CAD build for the part. Positions are in the model's coordinates, mm. A direction names the side the tool comes from. Round coordinates to 2 decimals unless told otherwise and drop trailing zeros. Loops run counter-clockwise (first coordinate to the right, second up) from the corner with the lowest first, then second, coordinate; pieces in that order, holes last. Notation, with made-up numbers: (46, -17.75) - (104, -17.75) arc R23 ccw to (104, 17.25) - close; hole circle Ø5 at (79.5, 59). An arc over 180 degrees is marked (long way). One line per question, with ' | ' between items.
```python
from build123d import *

# Parameters (mm, degrees)
F1_DEPTH        = 20
F2_DEPTH        = 8
F3_DEPTH        = 20
F4_R            = 5
F6_D            = 5.5
F7_R            = 5
F8_W            = 24.5
F8_H            = 5
F9_DEPTH        = 25
F11_D           = 5.5
F11_DEPTH       = 12
F11_CBORE_D     = 9.75
F11_CBORE_DEPTH = 2
F11_TIP         = 1.6523667023


with BuildPart() as f1:
    # F0 (on Top) → F1 (new body)
    with BuildSketch(Plane.XY):
        with BuildLine():
            Line((-7.3353787871, 29.9999998754), (-7.3353787871, 29.0893831246))
            ThreePointArc((-7.3353787871, 29.0893831246), (-23.6649673064, 18.4382568295), (-29.9999998754, 0))
            ThreePointArc((-29.9999998754, 0), (-21.2132033475, -21.2132033475), (0, -29.9999998754))
            ThreePointArc((0, -29.9999998754), (29.7714752963, -3.6958424215), (7.3353787871, 29.0893831246))
            Line((7.3353787871, 29.0893831246), (7.3353787871, 44.0893831246))
            Line((7.3353787871, 44.0893831246), (3.6676893936, 44.0893831246))
            Line((3.6676893936, 44.0893831246), (3.6676893936, 24.7294976599))
            ThreePointArc((3.6676893936, 24.7294976599), (0, -25), (-3.6676893936, 24.7294976599))
            Line((-3.6676893936, 24.7294976599), (-3.6676893936, 44.0893831246))
            Line((-3.6676893936, 44.0893831246), (-7.3353787871, 44.0893831246))
            Line((-7.3353787871, 44.0893831246), (-7.3353787871, 29.9999998754))
        make_face()
    extrude(amount=F1_DEPTH)

    # F0 (on Top) → F2 (join)
    with BuildSketch(Plane.XY):
        with BuildLine():
            Line((-7.3353787871, 29.9999998754), (-7.3353787871, 29.0893831246))
            ThreePointArc((-7.3353787871, 29.0893831246), (-23.6649673064, 18.4382568295), (-29.9999998754, 0))
            ThreePointArc((-29.9999998754, 0), (-21.2132033475, -21.2132033475), (0, -29.9999998754))
            ThreePointArc((0, -29.9999998754), (29.7714752963, -3.6958424215), (7.3353787871, 29.0893831246))
            Line((7.3353787871, 29.0893831246), (7.3353787871, 44.0893831246))
            Line((7.3353787871, 44.0893831246), (3.6676893936, 44.0893831246))
            Line((3.6676893936, 44.0893831246), (3.6676893936, 24.7294976599))
            ThreePointArc((3.6676893936, 24.7294976599), (0, -25), (-3.6676893936, 24.7294976599))
            Line((-3.6676893936, 24.7294976599), (-3.6676893936, 44.0893831246))
            Line((-3.6676893936, 44.0893831246), (-7.3353787871, 44.0893831246))
            Line((-7.3353787871, 44.0893831246), (-7.3353787871, 29.9999998754))
        make_face()
        with BuildLine():
            ThreePointArc((-29.9999998754, 0), (-23.6649673064, 18.4382568295), (-7.3353787871, 29.0893831246))
            Line((-7.3353787871, 29.0893831246), (-7.3353787871, 29.9999998754))
            Line((-7.3353787871, 29.9999998754), (-94.3353787871, 29.9999998754))
            ThreePointArc((-94.3353787871, 29.9999998754), (-96.4566991307, 29.1213202189), (-97.3353787871, 26.9999998754))
            Line((-97.3353787871, 26.9999998754), (-97.3353787871, -26.9999998754))
            ThreePointArc((-97.3353787871, -26.9999998754), (-96.4566991307, -29.1213202189), (-94.3353787871, -29.9999998754))
            Line((-94.3353787871, -29.9999998754), (-42.1122722328, -29.9999998754))
            Line((-42.1122722328, -29.9999998754), (-42.1122722328, 0))
            Line((-42.1122722328, 0), (-29.9999998754, 0))
        make_face()
        with BuildLine():
            ThreePointArc((0, -29.9999998754), (-21.2132033475, -21.2132033475), (-29.9999998754, 0))
            Line((-29.9999998754, 0), (-42.1122722328, 0))
            Line((-42.1122722328, 0), (-42.1122722328, -29.9999998754))
            Line((-42.1122722328, -29.9999998754), (0, -29.9999998754))
        make_face()
    extrude(amount=F2_DEPTH)

    # F0 (on Top) → F3 (join)
    with BuildSketch(Plane.XY):
        with BuildLine():
            ThreePointArc((0, -29.9999998754), (-21.2132033475, -21.2132033475), (-29.9999998754, 0))
            Line((-29.9999998754, 0), (-42.1122722328, 0))
            Line((-42.1122722328, 0), (-42.1122722328, -29.9999998754))
            Line((-42.1122722328, -29.9999998754), (0, -29.9999998754))
        make_face()
    extrude(amount=F3_DEPTH)

    # F4
    f4_edges = [f1.edges().sort_by_distance(p)[0] for p in [
        (5.501534, 44.089383, 0),
        (-5.501534, 44.089383, 0),
        (-5.501534, 44.089383, 20),
        (5.501534, 44.089383, 20),
    ]]
    fillet(f4_edges, radius=F4_R)

    # F6 (through all)
    with Locations(Plane.YZ.offset(7.3353787871)):
        with Locations((35.7856750488, 10)):
            Hole(F6_D / 2)

    # F7
    f7_edges = [f1.edges().sort_by_distance(p)[0] for p in [
        (-42.112272, 0, 14),
        (-30, 0, 14),
    ]]
    fillet(f7_edges, radius=F7_R)

    # F8 (on face) → F9 (cut)
    with BuildSketch(Plane(origin=(0, 0, 0), x_dir=(1, 0, 0), z_dir=(0, 0, -1))):
        with Locations((-28, 23.4999998754)):
            Rectangle(F8_W, F8_H)
    extrude(amount=-F9_DEPTH, mode=Mode.SUBTRACT)

    # F11
    with Locations(Plane.XZ.offset(29.9999998754)):
        with Locations((-35.5, 15), (-20.5, 15)):
            CounterBoreHole(F11_D / 2, F11_CBORE_D / 2, F11_CBORE_DEPTH, depth=F11_DEPTH)
            with Locations((0, 0, -(F11_DEPTH + F11_TIP / 2))):  # 118° drill point
                Cone(0, F11_D / 2, F11_TIP, mode=Mode.SUBTRACT)


solid = f1.part
```
(1) Cut at B-B, the plane x = 15. Write the cut outline in (y, z), then the cut area to 3 significant figures.
Results found:
outline: (-25.98, 0) - (-20, 0) - (-20, 20) - (-25.98, 20) - close; (20, 0) - (25.98, 0) - (25.98, 20) - (20, 20) - close | area: 239 mm²
(2) Probe L1, parallel to Z at x = -20.5, y = -27.3; L2, parallel to X at y = -19.9, z = 15; L3, parallel to X at y = -20.1, z = 15. List the from-to ranges inside material, lowest first.
Results found:
L1: z = 0 to 12.25, 17.75 to 20 | L2: x = -42.11 to -38.25, -32.75 to -23.25, -17.75 to -15.13, 15.13 to 22.45 | L3: x = -42.11 to -38.25, -32.75 to -23.25, -17.75 to -14.87, 14.87 to 22.27
(3) Two-plate mould, pull along Y, no slides. Class faces 1 (the face through (-40.686, -1.504, 14.084)), 2 (the face through (-32.753, -19.479, 15.121)), 3 (the face through (-28, -21, 10)): released by +Y, released by -Y, zero draft, split by the parting line, or undercut.
Results found:
face 1: released by +Y | face 2: zero draft | face 3: undercut
(4) Cut at C-C, the plane x = -85. Write the cut outline in (y, z).
Results found:
outline: (-30, 0) - (30, 0) - (30, 8) - (-30, 8) - close
(5) Cut at D-D, the plane y = 20. Write the cut outline in (x, z).
Results found:
outline: (-97.34, 0) - (-15, 0) - (-15, 20) - (-22.36, 20) - (-22.36, 8) - (-97.34, 8) - close; (15, 0) - (22.36, 0) - (22.36, 20) - (15, 20) - close
(6) Drop flat-ended pins along their axis: P1, Ø6, axis at x = -44.5, z = 14, coming from the +Y side; P2, Ø12, axis at x = -43, z = 14, coming from the -Y side; P3, Ø12, axis at y = 38.5, z = 13, coming from the +X side; P4, Ø8, axis at x = -20.5, z = 15.5, coming from the -Y side. Give the stop position or say it passes through.
Results found:
P1: stops at y = -2.6 | P2: stops at y = -30 | P3: stops at x = 7.34 | P4: stops at y = -28
(7) Tool access for faces 4 (the face through (-50, 30, 4)), 5 (the face through (-31.33, 1.253, 14.084)), 6 (the face through (-39.369, -29.014, 12.034)): list every direction of +Z, -Z, +X, -X, +Y, -Y with a clear straight run to the whole face (end or side of a thin tool).
Results found:
face 4: +Z, -Z, -X, +Y | face 5: +Z, -X, +Y | face 6: -Y
(8) Cut at A-A, the plane y = -12.5. Write the cut outline in (x, z), then the cut area to 3 significant figures.
Results found:
outline: (-97.34, 0) - (-21.65, 0) - (-21.65, 20) - (-42.11, 20) - (-42.11, 8) - (-97.34, 8) - close; (21.65, 0) - (27.27, 0) - (27.27, 20) - (21.65, 20) - close | area: 963 mm²
